The listing builds one solid part. Answer for the finished solid, in the listing's coordinates (mm). A direction names the side the tool comes from. Coordinates: 2 decimals unless noted, no trailing zeros. Loops run counter-clockwise (first coordinate to the right, second up) from the corner with the lowest first, then second, coordinate; pieces in that order, holes last. Notation, with made-up numbers: (84.5, -12.75) - (97.5, -12.75) arc R15 cw to (97.5, 2.25) - close; hole circle Ø9 at (-19.5, -40). An arc over 180 degrees is marked (long way). Return JSON: item names as keys, results as strings. Group by question number.
1. Section C-C (z = 0) is taken. Write down the section's boundary in (x, y).
2. Section A-A (x = 0) is taken. Write down the section's boundary in (y, z).
3. This flat-tipped pin is pushed along its axis until it touches: P1, Ø2, axis at x = -5, y = -166.5, coming from the -Z side. Where does it stop, or does it pass through?
4. The mould has two halves that part along Z. Classify faces 4 (the face through (-0.9, -167.04, -2.86)), 5 (the face through (-0.345, -162.521, 0.831)), 6 (the face through (0, -170, 0)): pulls with the +Z half, pulls with the -Z half, needs draft (parallel to the pull), parting line crosses it, or undercut.
5. Find the intervals of material crossed by line 1 along X through (y, z) = (-163.1, 0); line 2 along X through (y, z) = (-162.8, 3.25); line 3 along Y through (x, z) = (2.75, -6.5), in increasing order.
6. Section D-D (z = -6.5) is taken. Write down the section's boundary in (x, y), and give its area (4 significant figures).
7. Section B-B (y = -161.75) is taken. Write down the section's boundary in (x, z), and give its area (3 significant figures).
8. Which of the six approach directions +Z, -Z, +X, -X, +Y, -Y give full straight-line access (tool end or side, diameter ignored) to faces 1 (the face through (0, -162.5, -7.1)), 2 (the face through (-2.3, -164, 2.3)), 3 (the face through (0, -164, 0))?
```python
from build123d import *

# Parameters (mm, degrees)
SKETCH1_R               = 11.000723037
SKETCH1_R_2             = 0.9
SKETCH1_R_3             = 0.6
DISCO_APONEUROSIS_DEPTH = 3


with BuildPart() as part:
    # Sketch1 → Disco_aponeurosis (new body)
    with BuildSketch(Plane(origin=(0, -164, 0), x_dir=(1, 0, 0), z_dir=(0, 1, 0))):
        with Locations(Location((0, 0, 0), (0, 0, 270))):
            Circle(SKETCH1_R)
        with Locations(Location((0, 0, 0), (0, 0, 270))):
            Circle(SKETCH1_R_2, mode=Mode.SUBTRACT)
        with Locations(Location((0, 6.5, 0), (0, 0, 270))):
            Circle(SKETCH1_R_3, mode=Mode.SUBTRACT)
        with Locations(Location((-5.63, -3.25, 0), (0, 0, 270))):
            Circle(SKETCH1_R_3, mode=Mode.SUBTRACT)
        with Locations(Location((5.63, -3.25, 0), (0, 0, 270))):
            Circle(SKETCH1_R_3, mode=Mode.SUBTRACT)
    extrude(amount=DISCO_APONEUROSIS_DEPTH)

    # Sketch2 → Boca_tendon (revolve)
    with BuildSketch(Plane.XY, mode=Mode.PRIVATE) as boca_tendon_sk:
        Polygon((0, -164), (3, -164), (3, -170), (1.2, -170), (0, -170), align=None)
    revolve(boca_tendon_sk.sketch.rotate(Axis((0, -174, 0), (0, 1, 0)), 90), axis=Axis((0, -174, 0), (0, 1, 0)))


solid = part.part
```
The answers:
{
 "1": {"outline": "(-11, -164) - (-3, -164) - (-3, -170) - (3, -170) - (3, -164) - (11, -164) - (11, -161) - (0.9, -161) - (0.9, -164) - (-0.9, -164) - (-0.9, -161) - (-11, -161) - close"},
 "2": {"outline": "(-170, -3) - (-164, -3) - (-164, -5.9) - (-161, -5.9) - (-161, -0.9) - (-164, -0.9) - (-164, 0.9) - (-161, 0.9) - (-161, 11) - (-164, 11) - (-164, 3) - (-170, 3) - close; (-164, -11) - (-161, -11) - (-161, -7.1) - (-164, -7.1) - close"},
 "3": {"P1": "passes through"},
 "4": {"face 4": "parting line crosses it", "face 5": "undercut", "face 6": "needs draft"},
 "5": {"line 1": "x = -11 to -0.9, 0.9 to 11", "line 2": "x = -10.51 to -6.23, -5.03 to 5.03, 6.23 to 10.51", "line 3": "y = -164 to -161"},
 "6": {"outline": "(-8.88, -164) - (-0.6, -164) - (-0.6, -161) - (-8.88, -161) - close; (0.6, -164) - (8.88, -164) - (8.88, -161) - (0.6, -161) - close", "area": "49.65 mm2"},
 "7": {"outline": "circle Ø22 at (0, 0); hole circle Ø1.2 at (-5.63, 3.25); hole circle Ø1.8 at (0, 0); hole circle Ø1.2 at (0, -6.5); hole circle Ø1.2 at (5.63, 3.25)", "area": "374 mm2"},
 "8": {"face 1": "+Y, -Y", "face 2": "-Y", "face 3": "+Y"}
}
